Could you check a few things on this model? Use its own coordinates, in mm. A direction names the side the tool comes from. Round coordinates to 2 decimals unless told otherwise and drop trailing zeros. Loops run counter-clockwise (first coordinate to the right, second up) from the corner with the lowest first, then second, coordinate; pieces in that order, holes last. Notation, with made-up numbers: M 24,46 L 34,46 A9 ccw 34,62 Z; hole C 63,-5 d11. An arc over 180 degrees is marked long. One line per item, written item: value. Start each with the question number.
Q1. Please list where these lines run through material, in increasing order: line 1 along X through (y, z) = (6, -26.5); line 2 along Z through (x, y) = (-145.5, 5); line 3 along Y through (x, z) = (187.5, -67).
Q2. Which directions (+Z, -Z, +X, -X, +Y, -Y) give clear straight access to the entire face, cutting with the end or side of a thin tool? Please do faces 5 (the face through (-154, 10, -115)), 6 (the face through (100, 24, 2)), 7 (the face through (191.49, 9.4, -8.53)), 8 (the face through (-119.186, 5.553, 11.47)).
Q3. Imagine slicing it at B-B (x = -42.5). Please give me the cut outline in (y, z).
Q4. Imagine slicing it at A-A (z = -57.5). Give the number of separate pieces and of enclosed holes in the cut face, then the cut area to 3 significant figures.
Q5. I'm going to push flat-ended pins straight in: pin 1 Ø11 at (x, y) = (-182.5, 9) entering from -Z; pin 2 Ø6 at (x, z) = (64, 33.5) entering from +Y; pin 3 Ø2 at (x, y) = (85.5, 4.5) entering from -Z. Where does each tip first touch, or does it pass through?
Q6. Thinking about a two-plate mould opening in Y: for faces 1 (the face through (1, 10, -35)), 2 (the face through (3, -10, -30)), 3 (the face through (119.186, 5.553, 11.47)), 4 (the face through (-210, 18, -2)), which applies, released by +Y, released by -Y, zero draft, split by the parting line, or undercut?
from build123d import *

# Parameters (mm, degrees)
ESTRUSIONE_ESTRUSIONE1_DEPTH  = 10
SCHIZZO4_W                    = 110
SCHIZZO4_H                    = 230
ESTRUSIONE_ESTRUSIONE2_DEPTH  = 30
ESTRUSIONE_ESTRUSIONE6_DEPTH  = 110
ESTRUSIONE_ESTRUSIONE7_DEPTH  = 110
TAGLIO_ESTRUSIONE1_DEPTH      = 411.357133016
TAGLIO_ESTRUSIONE1_DEPTH_BACK = 411.357133016
SCHIZZO12_R                   = 9
ESTRUSIONE_ESTRUSIONE8_DEPTH  = 10
SCHIZZO13_R                   = 9
TAGLIO_ESTRUSIONE2_DEPTH      = 210
TAGLIO_ESTRUSIONE3_START      = -20
SCHIZZO13_3_R                 = 9
TAGLIO_ESTRUSIONE3_DEPTH      = 210


with BuildPart() as part:
    # Schizzo3 → Estrusione-Estrusione1 (new body)
    with BuildSketch(Plane(origin=(0, 0, 0), x_dir=(1, 0, 0), z_dir=(0, 1, 0))):
        Polygon((-100, 115), (0, 265), (100, 115), (100, -115), (-100, -115), align=None)
    extrude(amount=ESTRUSIONE_ESTRUSIONE1_DEPTH)

    # Schizzo4 → Estrusione-Estrusione2 (add)
    with BuildSketch(Plane(origin=(0, 0, 0), x_dir=(1, 0, 0), z_dir=(0, 1, 0))):
        with Locations((-155, 0)):
            Rectangle(SCHIZZO4_W, SCHIZZO4_H)
    estrusione_estrusione2 = extrude(amount=ESTRUSIONE_ESTRUSIONE2_DEPTH)

    # Specchia1: Estrusione-Estrusione2 across plane
    add(estrusione_estrusione2.mirror(Plane(origin=(0, 0, 0), x_dir=(0, 0, 1), z_dir=(1, 0, 0))))

    # Schizzo7 → Estrusione-Estrusione6 (add)
    with BuildSketch(Plane(origin=(210, 0, 0), x_dir=(0, 0, -1), z_dir=(1, 0, 0))):
        Polygon((-115, 30), (-67.116126168, 36.704444838), (-28.045596082, 30), align=None)
    estrusione_estrusione6 = extrude(amount=-ESTRUSIONE_ESTRUSIONE6_DEPTH)

    # Schizzo2 → Estrusione-Estrusione7 (add)
    with BuildSketch(Plane(origin=(100, 0, 0), x_dir=(0, 0, -1), z_dir=(1, 0, 0))):
        with BuildLine():
            add(Edge.make_bspline(
                [(-115, 30), (-115.000210545, 29.992600645), (-113.422148564, 30.158475864), (-111.796644727, 30.283772029), (-107.814194843, 30.630338356), (-102.861879623, 30.987329262), (-96.305865405, 31.376231826), (-88.489318037, 31.675517587), (-79.430494503, 31.807742684), (-69.341391082, 31.683388701), (-58.419850102, 31.274503076), (-46.877369477, 30.644796944), (-34.896947284, 29.847039434), (-22.646613535, 28.937405028), (-10.282420858, 27.977069897), (2.053986621, 27.029846245), (14.24124297, 26.170492863), (26.177229823, 25.446707781), (37.774042318, 24.895496731), (48.941874013, 24.516768377), (59.573909852, 24.266890816), (69.552699105, 24.140231832), (78.754080602, 24.115655421), (87.066553377, 24.222109148), (94.380340607, 24.454254196), (100.623442659, 24.835372596), (105.733457905, 25.450246293), (109.757791111, 26.267165094), (112.584447535, 27.347686718), (114.544522218, 28.409436669), (115.019506308, 29.606391564), (114.971300063, 30.713259492), (114.252481427, 32.105291566), (112.489642477, 33.883468186), (109.692003391, 35.61309624), (105.909966736, 37.265146946), (101.131610144, 38.854984679), (95.405801052, 40.36655429), (88.783353126, 41.751140678), (81.322054125, 42.956355889), (73.073722079, 43.933595569), (64.094685163, 44.671576526), (54.449786097, 45.162759351), (44.224155903, 45.437556505), (33.519437101, 45.505243934), (22.451785091, 45.379017652), (11.14328681, 45.063940096), (-0.28571179, 44.551548305), (-11.723358771, 43.840961212), (-23.065724405, 42.92819664), (-34.215267516, 41.845440169), (-45.069232514, 40.620473007), (-55.523547672, 39.302812034), (-65.469499205, 37.938342947), (-74.795963084, 36.558195732), (-83.315166316, 35.270519644), (-91.058717697, 33.948165881), (-97.854142359, 32.926071265), (-103.726595065, 31.930242691), (-108.212226347, 31.145720718), (-111.912932633, 30.508420978), (-113.462111319, 30.226412439), (-114.999791168, 30.00733917), (-115, 30)],
                knots=[0, 0, 0, 0, 0.001588889, 0.006329218, 0.014202456, 0.025172808, 0.039173483, 0.056060631, 0.075578924, 0.097363607, 0.120926258, 0.145825281, 0.171670912, 0.198108537, 0.224790184, 0.25139058, 0.277643491, 0.30332675, 0.328257458, 0.352272548, 0.375156062, 0.396620664, 0.416422729, 0.43430442, 0.45005468, 0.463465465, 0.474478994, 0.483169222, 0.489678354, 0.494104066, 0.496910015, 0.497289785, 0.501214273, 0.50645795, 0.513356957, 0.522168632, 0.53296597, 0.545689209, 0.560220779, 0.576438923, 0.594258689, 0.613600245, 0.634342386, 0.656331109, 0.679351894, 0.703152303, 0.727478208, 0.752070739, 0.776691164, 0.801140184, 0.825214387, 0.848697424, 0.871352858, 0.892947449, 0.913230871, 0.931955467, 0.948342069, 0.963693004, 0.976235918, 0.986320059, 0.993788799, 0.998424035, 1, 1, 1, 1], degree=3))
        make_face()
    estrusione_estrusione7 = extrude(amount=ESTRUSIONE_ESTRUSIONE7_DEPTH)

    # Specchia2: Estrusione-Estrusione6, Estrusione-Estrusione7 across plane
    add(estrusione_estrusione6.mirror(Plane(origin=(0, 0, 0), x_dir=(0, 0, 1), z_dir=(1, 0, 0))))
    add(estrusione_estrusione7.mirror(Plane(origin=(0, 0, 0), x_dir=(0, 0, 1), z_dir=(1, 0, 0))))

    # Schizzo12 → Taglio-Estrusione1 (cut, two sides: drawn at the far end of the back side and taken through both)
    with BuildSketch(Plane(origin=(100, 0, 0), x_dir=(0, 0, -1), z_dir=(1, 0, 0)).offset(-TAGLIO_ESTRUSIONE1_DEPTH_BACK)):
        with Locations((57.5, 34.659164248)):
            Circle(SCHIZZO12_R)
    extrude(amount=TAGLIO_ESTRUSIONE1_DEPTH + TAGLIO_ESTRUSIONE1_DEPTH_BACK, mode=Mode.SUBTRACT)

    # Schizzo14 → Estrusione-Estrusione8 (add)
    with BuildSketch(Plane.XZ):
        Polygon((-210, 115), (210, 115), (210, -115), (100, -115), (0, -265), (-100, -115), (-210, -115), align=None)
    extrude(amount=ESTRUSIONE_ESTRUSIONE8_DEPTH)

    # Schizzo13 → Taglio-Estrusione2 (cut)
    with BuildSketch(Plane.XY.offset(115)):
        with Locations((-127.5, 9)):
            Circle(SCHIZZO13_R)
    taglio_estrusione2 = extrude(amount=-TAGLIO_ESTRUSIONE2_DEPTH, mode=Mode.SUBTRACT)

    # Schizzo13<3> → Taglio-Estrusione3 (cut)
    with BuildSketch(Plane.XY.offset(115).offset(TAGLIO_ESTRUSIONE3_START)):
        with Locations((-182.5, 9)):
            Circle(SCHIZZO13_3_R)
    taglio_estrusione3 = extrude(amount=-TAGLIO_ESTRUSIONE3_DEPTH, mode=Mode.SUBTRACT)

    # Specchia3: Taglio-Estrusione2, Taglio-Estrusione3 across plane
    add(taglio_estrusione2.mirror(Plane(origin=(0, 0, 0), x_dir=(0, 0, 1), z_dir=(1, 0, 0))), mode=Mode.SUBTRACT)
    add(taglio_estrusione3.mirror(Plane(origin=(0, 0, 0), x_dir=(0, 0, 1), z_dir=(1, 0, 0))), mode=Mode.SUBTRACT)


solid = part.part
Report:
1. line 1: x = -210 to -190.99, -174.01 to -135.99, -119.01 to 119.01, 135.99 to 174.01, 190.99 to 210
1. line 2: z = -115 to 115
1. line 3: y = -10 to 1.52, 16.48 to 44.42
2. face 5: -Z, -X, +Y, -Y
2. face 6: +Z, -Z, +Y
2. face 7: -Z
2. face 8: +Z
3. outline: M -10,-201.25 L 10,-201.25 L 10,115 L -10,115 Z
4. separate pieces: 3
4. enclosed holes: 4
4. area: 11,100 mm²
5. pin 1: stops at z = 95
5. pin 2: stops at y = 10
5. pin 3: stops at z = -138.25
6. face 1: released by +Y
6. face 2: released by -Y
6. face 3: undercut
6. face 4: zero draft
